```python
from build123d import *

# Parameters (mm, degrees)
F2_DEPTH    = 9.525
F3_DEPTH    = 19.05
F4_T1_DEPTH = 31.861787518
F5_R        = 5.08


# Not quite as in the source:
# - a fillet or chamfer that OpenCascade refuses, or shapes differently, is made with other operations: its cross-section is extruded or revolved along the edge and cut away or added


with BuildPart() as f2:
    # F0 (on Top) → F2 (new body, symmetric)
    with BuildSketch(Plane.XY):
        with BuildLine():
            Line((0, 3.175), (0, 0))
            Line((0, 0), (19.05, 0))
            Line((19.05, 0), (19.05, -57.5181780653))
            ThreePointArc((19.05, -57.5181780653), (18.4056155347, -58.7951625359), (16.9955882353, -59.0354617085))
            ThreePointArc((16.9955882353, -59.0354617085), (9.0004674941, -57.9174166081), (1.0583333333, -59.3646503438))
            ThreePointArc((1.0583333333, -59.3646503438), (0.2913116778, -59.944816145), (0, -60.8613596973))
            ThreePointArc((0, -60.8613596973), (0.6709564477, -62.1575480195), (2.1166666667, -62.3580690508))
            ThreePointArc((2.1166666667, -62.3580690508), (10.0201305345, -61.0925159656), (17.859375, -62.708873578))
            ThreePointArc((17.859375, -62.708873578), (20.8248789571, -62.3981407308), (22.225, -59.7655698035))
            Line((22.225, -59.7655698035), (22.225, 3.175))
            Line((22.225, 3.175), (0, 3.175))
        make_face()
    extrude(amount=F2_DEPTH, both=True)

    # F1 (on Right) → F3 (join, through all)
    with BuildSketch(Plane.YZ):
        with BuildLine():
            Line((-6.6244696296, -9.525), (0, -9.525))
            Line((0, -9.525), (0, 0))
            ThreePointArc((0, 0), (-1.8189392592, -5.8010607408), (-6.6244696296, -9.525))
        make_face()
        with BuildLine():
            ThreePointArc((-6.6244696296, 9.525), (-1.8189392592, 5.8010607408), (0, 0))
            Line((0, 0), (0, 9.525))
            Line((0, 9.525), (-6.6244696296, 9.525))
        make_face()
    extrude(amount=F3_DEPTH)

    # F4: fillet of radius 1.5875 on 2 edges, made by hand

    # F4_s2 → F4_t1 (cut)
    with BuildSketch(Plane.YZ.offset(-12.811787518)):
        with BuildLine():
            ThreePointArc((-1.4997546224, 9.525), (-2.9528486536, 8.5767761426), (-2.6700580518, 6.8648648649))
            ThreePointArc((-2.6700580518, 6.8648648649), (-4.4890794666, 8.4300806819), (-6.6244696296, 9.525))
            Line((-6.6244696296, 9.525), (-1.4997546224, 9.525))
        make_face()
        with BuildLine():
            ThreePointArc((-1.4997546224, -9.525), (-2.9528486536, -8.5767761426), (-2.6700580518, -6.8648648649))
            ThreePointArc((-2.6700580518, -6.8648648649), (-4.4890794666, -8.4300806819), (-6.6244696296, -9.525))
            Line((-6.6244696296, -9.525), (-1.4997546224, -9.525))
        make_face()
    extrude(amount=F4_T1_DEPTH, mode=Mode.SUBTRACT)

    # F5
    f5_edges = [f2.edges().sort_by_distance(p)[0] for p in [
        (22.225, 3.175, -4.7625),
        (22.225, 3.175, 4.7625),
    ]]
    fillet(f5_edges, radius=F5_R)


solid = f2.part
```
Can you work these out from the model? Positions are in its coordinate system, mm. A direction names the side the tool comes from. Give positions to 0.01 mm unless a question says otherwise; leave off trailing zeros. Write each loop counter-clockwise with the first axis right and the second up, starting at its lowest first coordinate (ties: lowest second). Pieces come first, ordered by that corner, then holes. Notation, with made-up numbers: (55.5, 59) - (107.5, 59) arc R11 ccw to (107.5, 64) - close; hole circle Ø4 at (10, 9). An arc over 180 degrees is marked (long way). Write item = value, one per line. Start each with the question number.
1. Imagine slicing it at A-A (x = 6.5). Please give me the cut outline in (y, z) (1 decimal).
2. Imagine slicing it at D-D (y = -16). Please give me the cut outline in (x, z) (3 decimals), and give its area (3 significant figures).
3. For pin 1 (8 mm diameter, centred on x = 17, y = -5, fed in from +Z) (3 decimals); pin 2 (2 mm diameter, centred on x = 4.5, z = -5.5, fed in from -Y); pin 3 (1 mm diameter, centred on y = -6, z = 6.5, fed in from -X), each with a flat end and sliding along its axis, tell me the tip position at first contact or that it passes through.
4. On a 3-axis mill with a long thin cutter (end or side, diameter ignored), from which of +Z, -Z, +X, -X, +Y, -Y can I reach the whole of each face in a straight line? I mean faces 1 (the face through (9.114, -57.915, 0.133)), 2 (the face through (9.392, -2.942, -8.6)), 3 (the face through (22.225, -31, 0)). Say none if no direction works.
5. Thinking about a two-plate mould opening in X: for faces 4 (the face through (9, 3.175, 0)), 5 (the face through (9.91, -61.09, 0.13)), 6 (the face through (20.79, -62.42, 0.13)), which applies, released by +X, released by -X, zero draft, split by the parting line, or undercut?
6. Please list where these lines run through material, in increasing order: line 1 (X direction, y = -45, z = 0.5) (3 decimals); line 2 (Y direction, x = 8, z = -5.75) (3 decimals); line 3 (Y direction, x = 5.5, z = -6.25) (1 decimal).
7. Imagine slicing it at C-C (x = 11.5). Please give me the cut outline in (y, z) (1 decimal), and give its area (3 significant figures).
Worked answers:
q1.outline = (-61.3, -9.5) - (-58.1, -9.5) - (-58.1, 9.5) - (-61.3, 9.5) - close; (-2.7, -6.9) arc R1.6 ccw to (-1.5, -9.5) - (3.2, -9.5) - (3.2, 9.5) - (-1.5, 9.5) arc R1.6 ccw to (-2.7, 6.9) arc R10.2 cw to start
q2.outline = (19.05, -9.525) - (22.225, -9.525) - (22.225, 9.525) - (19.05, 9.525) - close
q2.area = 60.5 mm2
q3.pin_1 = 9.525
q3.pin_2 = -61.92
q3.pin_3 = 19.05
q4.face_1 = +Z, -Z
q4.face_2 = -X
q4.face_3 = +Z, -Z, +X, +Y, -Y
q5.face_4 = zero draft
q5.face_5 = undercut
q5.face_6 = split by the parting line
q6.line_1 = 19.05 to 22.225
q6.line_2 = -61.139 to -57.958, -1.784 to 3.175
q6.line_3 = -61.5 to -58.2, -2.1 to 3.2
q7.outline = (-61.2, -9.5) - (-58, -9.5) - (-58, 9.5) - (-61.2, 9.5) - close; (-2.7, -6.9) arc R1.6 ccw to (-1.5, -9.5) - (3.2, -9.5) - (3.2, 9.5) - (-1.5, 9.5) arc R1.6 ccw to (-2.7, 6.9) arc R10.2 cw to start
q7.area = 148 mm2
